```python
from build123d import *

# Parameters (mm, degrees)
F1_DEPTH  = 17
F3_T      = -2
F2_R      = 8.5
F4_DEPTH  = 2
F5_R      = 1
F6_DEPTH  = 15
F7_R      = 1
F8_DEPTH  = 7
F11_DEPTH = 10
F12_DEPTH = 8
F13_DEPTH = 2


with BuildPart() as f1:
    # F0 (on Top) → F1 (new body)
    with BuildSketch(Plane.XY):
        with BuildLine():
            Line((-12.5, 17.5), (-37.5, 17.5))
            ThreePointArc((-37.5, 17.5), (-39.6213203436, 16.6213203436), (-40.5, 14.5))
            Line((-40.5, 14.5), (-40.5, -17.5))
            Line((-40.5, -17.5), (-40.5, -35.5))
            ThreePointArc((-40.5, -35.5), (-39.6213203436, -37.6213203436), (-37.5, -38.5))
            Line((-37.5, -38.5), (55.5, -38.5))
            ThreePointArc((55.5, -38.5), (57.6213203436, -37.6213203436), (58.5, -35.5))
            Line((58.5, -35.5), (58.5, -17.5))
            Line((58.5, -17.5), (40.5, -17.5))
            Line((40.5, -17.5), (40.5, 17.5))
            Line((40.5, 17.5), (40.5, 42.5))
            ThreePointArc((40.5, 42.5), (39.6213203436, 44.6213203436), (37.5, 45.5))
            Line((37.5, 45.5), (-6.5, 45.5))
            ThreePointArc((-6.5, 45.5), (-8.6213203436, 44.6213203436), (-9.5, 42.5))
            Line((-9.5, 42.5), (-9.5, 20.5))
            ThreePointArc((-9.5, 20.5), (-10.3786796564, 18.3786796564), (-12.5, 17.5))
        make_face()
        with BuildLine():
            Line((55.5, 45.5), (37.5, 45.5))
            ThreePointArc((37.5, 45.5), (39.6213203436, 44.6213203436), (40.5, 42.5))
            Line((40.5, 42.5), (40.5, 17.5))
            Line((40.5, 17.5), (40.5, -17.5))
            Line((40.5, -17.5), (58.5, -17.5))
            Line((58.5, -17.5), (58.5, 42.5))
            ThreePointArc((58.5, 42.5), (57.6213203436, 44.6213203436), (55.5, 45.5))
        make_face()
    extrude(amount=F1_DEPTH)

    # F3
    f3_openings = [f1.faces().sort_by_distance(p)[0] for p in [
        (12.966173, 0.233802, 17),
    ]]
    offset(amount=F3_T, openings=f3_openings)

    # F2 (on Top) → F4 (cut, through all)
    with BuildSketch(Plane.XY):
        with BuildLine():
            add(Edge.make_bspline(
                [(-25, 10.5), (-39.7224318643, 10.5), (-32.3612159322, -3.75), (-25, -18), (-17.6387840678, -3.75), (-10.2775681357, 10.5), (-25, 10.5)],
                knots=[0, 0, 0, 2.0943951024, 2.0943951024, 4.1887902048, 4.1887902048, 6.2831853072, 6.2831853072, 6.2831853072], degree=2, weights=[1, 0.5, 1, 0.5, 1, 0.5, 1]))
        make_face()
        with BuildLine():
            add(Edge.make_bspline(
                [(24, -4.5), (38.7224318643, -4.5), (31.3612159322, 9.75), (24, 24), (16.6387840678, 9.75), (9.2775681357, -4.5), (24, -4.5)],
                knots=[0, 0, 0, 2.0943951024, 2.0943951024, 4.1887902048, 4.1887902048, 6.2831853072, 6.2831853072, 6.2831853072], degree=2, weights=[1, 0.5, 1, 0.5, 1, 0.5, 1]))
        make_face()
        with Locations((-0.5, -6)):
            Circle(F2_R)
    extrude(amount=F4_DEPTH, mode=Mode.SUBTRACT)

    # F5 (on face) → F6 (join, through all)
    with BuildSketch(Plane.XY.offset(2)):
        with BuildLine():
            ThreePointArc((51.5, 41), (52.232233047, 39.232233047), (54, 38.5))
            Line((54, 38.5), (56.5, 38.5))
            Line((56.5, 38.5), (56.5, 43.5))
            Line((56.5, 43.5), (51.5, 43.5))
            Line((51.5, 43.5), (51.5, 41))
        make_face()
        with Locations((54, 41)):
            Circle(F5_R, mode=Mode.SUBTRACT)
        with BuildLine():
            Line((-2.5, 43.5), (-7.5, 43.5))
            Line((-7.5, 43.5), (-7.5, 38.5))
            Line((-7.5, 38.5), (-7.5, 20.5))
            Line((-7.5, 20.5), (-12.5, 15.5))
            Line((-12.5, 15.5), (-7.5, 15.5))
            ThreePointArc((-7.5, 15.5), (-3.9644660941, 16.9644660941), (-2.5, 20.5))
            Line((-2.5, 20.5), (-2.5, 43.5))
        make_face()
        with Locations((-5, 41)):
            Circle(F5_R, mode=Mode.SUBTRACT)
        with BuildLine():
            Line((56.5, -31.5), (54, -31.5))
            ThreePointArc((54, -31.5), (52.232233047, -32.232233047), (51.5, -34))
            Line((51.5, -34), (51.5, -36.5))
            Line((51.5, -36.5), (56.5, -36.5))
            Line((56.5, -36.5), (56.5, -31.5))
        make_face()
        with Locations((54, -34)):
            Circle(F5_R, mode=Mode.SUBTRACT)
        with BuildLine():
            Line((-33.5, -36.5), (-33.5, -34))
            ThreePointArc((-33.5, -34), (-34.232233047, -32.232233047), (-36, -31.5))
            Line((-36, -31.5), (-38.5, -31.5))
            Line((-38.5, -31.5), (-38.5, -36.5))
            Line((-38.5, -36.5), (-33.5, -36.5))
        make_face()
        with Locations((-36, -34)):
            Circle(F5_R, mode=Mode.SUBTRACT)
    extrude(amount=F6_DEPTH)

    # F7 (on face) → F8 (cut, through all)
    with BuildSketch(Plane(origin=(-9.5, 0, 0), x_dir=(0, -1, 0), z_dir=(-1, 0, 0))):
        with Locations((-26.5, 17)):
            Circle(F7_R)
        with Locations((-36.5, 17)):
            Circle(F7_R)
    extrude(amount=-F8_DEPTH, mode=Mode.SUBTRACT)

    # F10 (on face) → F11 (join)
    with BuildSketch(Plane(origin=(0, 0, 0), x_dir=(1, 0, 0), z_dir=(0, 0, -1))):
        with BuildLine():
            Line((55.5, 38.5), (-37.5, 38.5))
            ThreePointArc((-37.5, 38.5), (-39.6213203436, 37.6213203436), (-40.5, 35.5))
            Line((-40.5, 35.5), (-40.5, 14.5))
            Line((-40.5, 14.5), (-0.5, 14.5))
            Line((-0.5, 14.5), (58.5, 14.5))
            Line((58.5, 14.5), (58.5, 35.5))
            ThreePointArc((58.5, 35.5), (57.6213203436, 37.6213203436), (55.5, 38.5))
        make_face()
    extrude(amount=F11_DEPTH)

    # F9 (on face) → F12 (cut)
    with BuildSketch(Plane(origin=(0, 0, 0), x_dir=(1, 0, 0), z_dir=(0, 0, -1))):
        with BuildLine():
            Line((56.4999997616, 16.5000002384), (56.4999997616, 35.5))
            ThreePointArc((56.4999997616, 35.5), (56.2071066126, 36.2071066126), (55.5, 36.4999997616))
            Line((55.5, 36.4999997616), (-37.5, 36.4999997616))
            ThreePointArc((-37.5, 36.4999997616), (-38.2071066126, 36.2071066126), (-38.4999997616, 35.5))
            Line((-38.4999997616, 35.5), (-38.4999997616, 16.5000002384))
            Line((-38.4999997616, 16.5000002384), (56.4999997616, 16.5000002384))
        make_face()
    extrude(amount=F12_DEPTH, mode=Mode.SUBTRACT)

    # F9 (on face) → F13 (cut)
    with BuildSketch(Plane(origin=(0, 0, 0), x_dir=(1, 0, 0), z_dir=(0, 0, -1))):
        with BuildLine():
            Line((56.4999997616, 16.5000002384), (56.4999997616, 35.5))
            ThreePointArc((56.4999997616, 35.5), (56.2071066126, 36.2071066126), (55.5, 36.4999997616))
            Line((55.5, 36.4999997616), (-37.5, 36.4999997616))
            ThreePointArc((-37.5, 36.4999997616), (-38.2071066126, 36.2071066126), (-38.4999997616, 35.5))
            Line((-38.4999997616, 35.5), (-38.4999997616, 16.5000002384))
            Line((-38.4999997616, 16.5000002384), (56.4999997616, 16.5000002384))
        make_face()
    extrude(amount=-F13_DEPTH, mode=Mode.SUBTRACT)


solid = f1.part
```
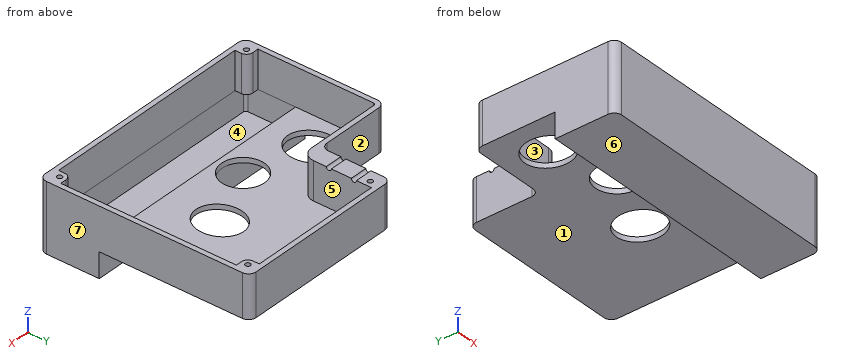
Part model, mm, in its own coordinate system. Face numbers are marked on the shaded views. A direction names the side the tool comes from. Round coordinates to 2 decimals unless told otherwise and drop trailing zeros. Loops run counter-clockwise (first coordinate to the right, second up) from the corner with the lowest first, then second, coordinate; pieces in that order, holes last. Notation, with made-up numbers: (53.5, 79) -> (63.5, 79) arc R18 ccw to (63.5, 94) -> close; hole circle Ø6 at (-13, 74). An arc over 180 degrees is marked (long way). Use one line per item in the form item = value. Start each with the question number.
Item 1: Tool access for the marked faces 1, 2 and 3: list every direction of +Z, -Z, +X, -X, +Y, -Y with a clear straight run to the whole face (end or side of a thin tool).
Item 2: Drop flat-ended pins along their axis: pin 1 Ø1 at (x, z) = (-29, 9.5) entering from +Y; pin 2 Ø2 at (x, y) = (-5.5, 41.5) entering from +Z; pin 3 Ø4 at (y, z) = (23, 13.5) entering from -X; pin 4 Ø5 at (x, z) = (31, -4) entering from +Y. Give the stop position or say it passes through.
Item 3: Band-saw the part on B-B (y = 33). List the corners of the cut face in (x, z).
Item 4: Band-saw the part on C-C (z = -6). List the corners of the cut face in (x, y).
Item 5: Band-saw the part on A-A (x = 12). List the corners of the cut face in (y, z).
Item 6: Two-plate mould, pull along X, no slides. Class the marked faces 4, 5, 6 and 7: released by +X, released by -X, zero draft, split by the parting line, or undercut.
Item 7: Band-saw the part on D-D (z = 9.5). Give the number of separate pieces and of enclosed holes in the cut face, plus the area to 3 significant figures.
Item 8: Drill centre lines: line 1 along Y through (x, z) = (54, 13.25); line 2 along Y through (x, z) = (-36, 11.75); line 3 along Y through (x, z) = (-27, 11). Where is each one in solid material? Low to high.
Data:
q1.face_1 = -Z, +X, -X, +Y
q1.face_2 = +Z, -Z, -X, +Y
q1.face_3 = +Z
q2.pin_1 = 17.5
q2.pin_2 = 17
q2.pin_3 = -9.5
q2.pin_4 = -14.5
q3.outline = (-9.5, 0) -> (58.5, 0) -> (58.5, 17) -> (56.5, 17) -> (56.5, 2) -> (-2.5, 2) -> (-2.5, 17) -> (-9.5, 17) -> close
q4.outline = (-40.5, -35.5) arc R3 ccw to (-37.5, -38.5) -> (55.5, -38.5) arc R3 ccw to (58.5, -35.5) -> (58.5, -14.5) -> (-40.5, -14.5) -> close; hole (-38.5, -35.5) arc R1 ccw to (-37.5, -36.5) -> (55.5, -36.5) arc R1 ccw to (56.5, -35.5) -> (56.5, -16.5) -> (-38.5, -16.5) -> close
q5.outline = (-38.5, -10) -> (-14.5, -10) -> (-14.5, 0) -> (45.5, 0) -> (45.5, 17) -> (43.5, 17) -> (43.5, 2) -> (-16.5, 2) -> (-16.5, -8) -> (-36.5, -8) -> (-36.5, 17) -> (-38.5, 17) -> close
q6.face_4 = undercut
q6.face_5 = undercut
q6.face_6 = zero draft
q6.face_7 = released by +X
q7.separate_pieces = 1
q7.enclosed_holes = 5
q7.area = 902 mm^2
q8.line_1 = -38.5 to -35, -33 to -31.5, 38.5 to 40, 42 to 45.5
q8.line_2 = -38.5 to -35, -33 to -31.5, 15.5 to 17.5
q8.line_3 = -38.5 to -36.5, 15.5 to 17.5
